Geometry check sheet. Reference: drawing and pictorial views, mm from the part's lowest x, y, z. A direction names the side the tool comes from. Give positions to 0.01 mm unless a question says otherwise; leave off trailing zeros. Order: outer loops, then holes, each group sorted by start corner. A loop starts at its lowest first (then second) coordinate and runs counter-clockwise, first axis right, second up. Notation, with made-up numbers: M -29.5,63 L 10.5,63 A6 cw 10.5,68 Z; hole C -39,40.5 d2. An arc over 180 degrees is marked long. Use CSV: the item, a comma, the result in double quotes. Start each with the question number.
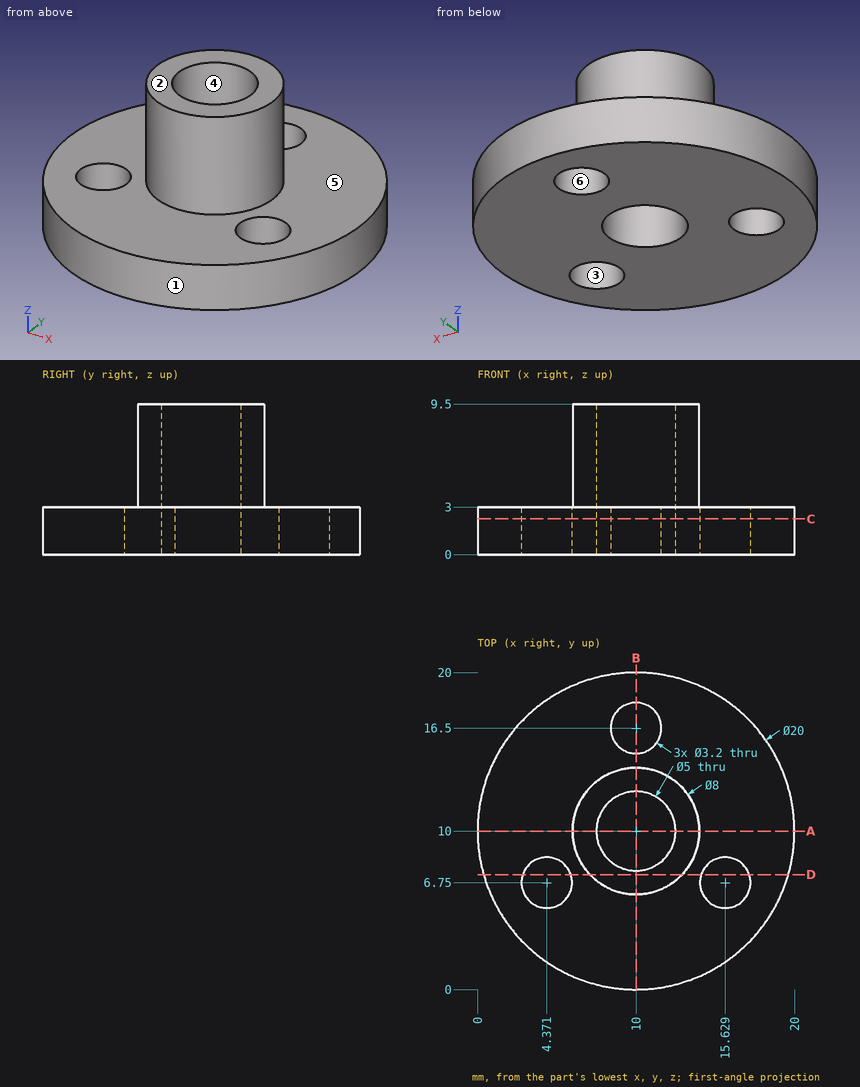
(1) Draft check along Y on the marked faces 1, 2, 3 and 4. Enter one of: +Y half, -Y half, draft (parallel to the pull), parting line (faces both ways), or undercut.
(2) Sectioned sample at B-B on x = 10. Record the cut outline in (y, z), then the cut area to 3 significant figures.
(3) Access from +Z, -Z, +X, -X, +Y, -Y to the whole of each face (thin tool, end or side, straight path). Record for the marked faces 5 and 6.
(4) Thickness scan on line 1 (Y direction, x = 10, z = 1); line 2 (Y direction, x = 10, z = 7.25); line 3 (X direction, y = 5.75, z = 0.75). Record the ranges inside material, lowest first.
(5) Sectioned sample at D-D on y = 7.25. Record the cut outline in (x, z) (1 decimal), then the cut area to 3 significant figures.
(6) Go/stop test with flat-tipped pins: P1, Ø2.5, axis at x = 15.63, y = 6.75, coming from the -Z side; P2, Ø1, axis at x = 15, y = 14.5, coming from the +Z side; P3, Ø4, axis at y = 5.5, z = 1, coming from the -X side. Record where each tip stops, or that it passes through.
(7) Sectioned sample at C-C on z = 2.25. Record the cut outline in (x, y).
(8) Sectioned sample at A-A on y = 10. Record the cut outline in (x, z).
Responses:
1,face 1,"parting line"
1,face 2,"draft"
1,face 3,"undercut"
1,face 4,"undercut"
2,outline,"M 0,0 L 7.5,0 L 7.5,9.5 L 6,9.5 L 6,3 L 0,3 Z; M 12.5,0 L 14.9,0 L 14.9,3 L 14,3 L 14,9.5 L 12.5,9.5 Z; M 18.1,0 L 20,0 L 20,3 L 18.1,3 Z"
2,area,"54.9 mm2"
3,face 5,"+Z"
3,face 6,"+Z, -Z"
4,line 1,"0 to 7.5, 12.5 to 14.9, 18.1 to 20"
4,line 2,"6 to 7.5, 12.5 to 14"
4,line 3,"0.95 to 3.12, 5.62 to 14.38, 16.88 to 19.05"
5,outline,"M 0.4,0 L 2.9,0 L 2.9,3 L 0.4,3 Z; M 5.9,0 L 14.1,0 L 14.1,3 L 12.9,3 L 12.9,9.5 L 7.1,9.5 L 7.1,3 L 5.9,3 Z; M 17.1,0 L 19.6,0 L 19.6,3 L 17.1,3 Z"
5,area,"77.2 mm2"
6,P1,"through"
6,P2,"z = 3"
6,P3,"x = 0.32"
7,outline,"C 10,10 d20; hole C 4.37,6.75 d3.2; hole C 10,10 d5; hole C 10,16.5 d3.2; hole C 15.63,6.75 d3.2"
8,outline,"M 0,0 L 7.5,0 L 7.5,9.5 L 6,9.5 L 6,3 L 0,3 Z; M 12.5,0 L 20,0 L 20,3 L 14,3 L 14,9.5 L 12.5,9.5 Z"
